Geometry check sheet. Reference: the model listing, model coordinates, mm. A direction names the side the tool comes from. Give positions to 0.01 mm unless a question says otherwise; leave off trailing zeros. Loops run counter-clockwise (first coordinate to the right, second up) from the corner with the lowest first, then second, coordinate; pieces in that order, holes last. Notation, with made-up numbers: (-22.5, 73) -> (-11.5, 73) arc R23 cw to (-11.5, 93) -> close; hole circle Ø11 at (-27.5, 0.5). An arc over 180 degrees is marked (long way). One line per item, written item: value. Start each with the question number.
(1) Sectioned sample at A-A, the plane z = 14.5. Record the cut outline in (x, y), then the cut area to 3 significant figures.
(2) Gauge pin test, flat ends, axial feed: pin 1 Ø3 at (x, z) = (2, -60) entering from +Y; pin 2 Ø1.8 at (x, y) = (4, -120) entering from +Z. Record the tip position at first contact, or that the pin passes through.
(3) Draft check along Z on faces 1 (the face through (3, 0, 62.25)), 2 (the face through (3, 93, -44.25)), 3 (the face through (3, -68, -62.25)). Enter one of: pulls with the +Z half, pulls with the -Z half, needs draft (parallel to the pull), parting line crosses it, or undercut.
(4) Tool access check on faces 4 (the face through (3, 102, -56.25)), 5 (the face through (3, -51, 59)), 6 (the face through (3, 93, 32.25)), 7 (the face through (3, -109, -56.25)), 8 (the face through (3, -51, -59)). Record the directions out of +Z, -Z, +X, -X, +Y, -Y that give a thin tool (end or side, any length) a straight path to the whole face; none if there is none.
(5) Sectioned sample at B-B, the plane x = 2.55. State how many separate pieces and enclosed holes the cut face has, then the cut area to 3 significant figures.
(6) Sectioned sample at C-C, the plane y = 40. Record the cut outline in (x, z).
(7) Scan lines: line 1 along Y through (x, z) = (3.3, -15); line 2 along Y through (x, z) = (4.9, -34); line 3 along Z through (x, y) = (3.6, -114.5). Record each from-to range of solid material in increasing order. Write a range as from..to.
from build123d import *

# Parameters (mm, degrees)
SKETCH1_W           = 112.5
SKETCH1_H           = 238
BOSS_EXTRUDE1_DEPTH = 6
SKETCH4_W           = 6
SKETCH4_H           = 22.5
BOSS_EXTRUDE2_DEPTH = 6
SKETCH5_W           = 6
SKETCH5_H           = 34
BOSS_EXTRUDE3_DEPTH = 6
SKETCH6_W           = 12
SKETCH6_H           = 6
CUT_EXTRUDE1_DEPTH  = 800
SKETCH7_W           = 6
SKETCH7_H           = 112.5
BOSS_EXTRUDE4_DEPTH = 8


with BuildPart() as part:
    # Sketch1 → Boss-Extrude1 (new body)
    with BuildSketch(Plane(origin=(0, 0, 0), x_dir=(0, 0, -1), z_dir=(1, 0, 0))):
        Rectangle(SKETCH1_W, SKETCH1_H)
    extrude(amount=BOSS_EXTRUDE1_DEPTH)

    # Sketch4 → Boss-Extrude2 (add)
    with BuildSketch(Plane.XZ.offset(119)):
        with Locations((3, -45)):
            Rectangle(SKETCH4_W, SKETCH4_H)
        with Locations((3, 0)):
            Rectangle(SKETCH4_W, SKETCH4_H)
        with Locations((3, 45)):
            Rectangle(SKETCH4_W, SKETCH4_H)
    extrude(amount=BOSS_EXTRUDE2_DEPTH)

    # Sketch5 → Boss-Extrude3 (add)
    with BuildSketch(Plane(origin=(0, 0, -56.25), x_dir=(-1, 0, 0), z_dir=(0, 0, -1))):
        with Locations((-3, -68)):
            Rectangle(SKETCH5_W, SKETCH5_H)
        with Locations((-3, 0)):
            Rectangle(SKETCH5_W, SKETCH5_H)
        with Locations((-3, 68)):
            Rectangle(SKETCH5_W, SKETCH5_H)
    boss_extrude3 = extrude(amount=BOSS_EXTRUDE3_DEPTH)

    # Mirror1: Boss-Extrude3 across plane
    add(boss_extrude3.mirror(Plane.XY))

    # Sketch6 → Cut-Extrude1 (cut)
    with BuildSketch(Plane(origin=(6, 0, 0), x_dir=(0, 0, -1), z_dir=(1, 0, 0))):
        with Locations((-38.25, 93)):
            Rectangle(SKETCH6_W, SKETCH6_H)
        with Locations((38.25, 93)):
            Rectangle(SKETCH6_W, SKETCH6_H)
    extrude(amount=-CUT_EXTRUDE1_DEPTH, mode=Mode.SUBTRACT)

    # Sketch7 → Boss-Extrude4 (add)
    with BuildSketch(Plane.XZ.offset(125)):
        with Locations((3, 0)):
            Rectangle(SKETCH7_W, SKETCH7_H)
    extrude(amount=BOSS_EXTRUDE4_DEPTH)


solid = part.part
Calculated:
1. outline: (0, -133) -> (6, -133) -> (6, -125) -> (0, -125) -> close; (0, -119) -> (6, -119) -> (6, 119) -> (0, 119) -> close
1. area: 1,480 mm2
2. pin 1: stops at y = 85
2. pin 2: stops at z = 56.25
3. face 1: pulls with the +Z half
3. face 2: undercut
3. face 3: pulls with the -Z half
4. face 4: -Z, +X, -X, +Y
4. face 5: +Z, +X, -X
4. face 6: +X, -X
4. face 7: -Z, +X, -X, -Y
4. face 8: -Z, +X, -X
5. separate pieces: 1
5. enclosed holes: 4
5. area: 29,200 mm2
6. outline: (0, -56.25) -> (6, -56.25) -> (6, 56.25) -> (0, 56.25) -> close
7. line 1: y = -133..-125, -119..119
7. line 2: y = -133..90, 96..119
7. line 3: z = -56.25..56.25
